Can you work these out from the model? Positions are in its coordinate system, mm. Face numbers are marked on the shaded views. A direction names the side the tool comes from. Give positions to 0.01 mm unless a question says otherwise; leave off trailing zeros. Order: outer loops, then holes, each group sorted by start corner. A loop starts at its lowest first (then second) coordinate and runs counter-clockwise, first axis right, second up. Notation, with made-up numbers: (17.25, 82.5) - (65.25, 82.5) arc R30 cw to (65.25, 112.5) - close; hole circle Ø1 at (-16.5, -23). An arc over 180 degrees is marked (long way). Return JSON: item names as keys, results as strings.
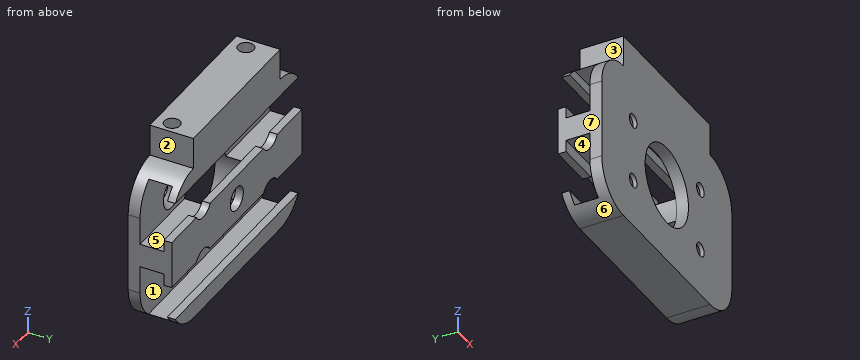
```python
from build123d import *
from build123d.topology import SkipClean

# Parameters (mm, degrees)
SKETCH1_R           = 9.999999259
SKETCH1_R_2         = 1.748202303
SKETCH1_R_3         = 1.748202071
BOSS_EXTRUDE1_DEPTH = 3
BOSS_EXTRUDE2_REACH = 65.317
BOSS_EXTRUDE3_DEPTH = 59.999998659
CUT_EXTRUDE1_START  = 18
SKETCH3_R           = 9.999999259
CUT_EXTRUDE1_DEPTH  = 18
SKETCH4_W           = 63.792856733
SKETCH4_H           = 41.767533566
CUT_EXTRUDE2_DEPTH  = 29
SKETCH5_R           = 2.99999956
CUT_EXTRUDE3_DEPTH  = 29
CHAMFER1_SIZE       = 2
CHAMFER2_SIZE       = 2
SKETCH6_R           = 3.748202071
SKETCH6_R_2         = 3.748202303
CUT_EXTRUDE4_DEPTH  = 3
SKETCH7_R           = 1.5
CUT_EXTRUDE5_DEPTH  = 2
SKETCH9_W           = 40.000000969
SKETCH9_H           = 2
BOSS_EXTRUDE4_DEPTH = 11
SKETCH10_W          = 40.000000969
SKETCH10_H          = 10.999999914
SKETCH10_R          = 2
BOSS_EXTRUDE5_DEPTH = 6
CUT_EXTRUDE6_START  = -3.945921595
SKETCH10_3_R        = 2
CUT_EXTRUDE6_DEPTH  = 3.945921595


with BuildPart() as part:
    # Sketch1 → Boss-Extrude1 (new body)
    with BuildSketch(Plane(origin=(0, 0, 0), x_dir=(1, 0, 0), z_dir=(0, 1, 0))):
        with BuildLine():
            Line((-19.999999553, -20.000000484), (20.000001416, -20.000000484))
            ThreePointArc((20.000001416, -20.000000484), (27.071068604, -17.071068441), (29.999999329, -10.000000708))
            Line((29.999999329, -10.000000708), (29.999999329, 9.999998845))
            ThreePointArc((29.999999329, 9.999998845), (27.071068411, 17.071066386), (20.000001416, 19.999998622))
            Line((20.000001416, 19.999998622), (-19.999999553, 19.999998622))
            ThreePointArc((-19.999999553, 19.999998622), (-27.071067207, 17.071066499), (-29.999999329, 9.999998845))
            Line((-29.999999329, 9.999998845), (-29.999999329, -10.000000708))
            ThreePointArc((-29.999999329, -10.000000708), (-27.071067207, -17.071068362), (-19.999999553, -20.000000484))
        make_face()
        with Locations(Location((0, 0, 0), (0, 0, 270))):
            Circle(SKETCH1_R, mode=Mode.SUBTRACT)
        with Locations(Location((15.500057023, 8.001796436, 0), (0, 0, 270))):
            Circle(SKETCH1_R_2, mode=Mode.SUBTRACT)
        with Locations(Location((-15.500057023, 8.001796436, 0), (0, 0, 270))):
            Circle(SKETCH1_R_2, mode=Mode.SUBTRACT)
        with Locations(Location((-15.500057023, -7.998204092, 0), (0, 0, 270))):
            Circle(SKETCH1_R_3, mode=Mode.SUBTRACT)
        with Locations(Location((15.500057023, -7.998204092, 0), (0, 0, 270))):
            Circle(SKETCH1_R_3, mode=Mode.SUBTRACT)
    extrude(amount=BOSS_EXTRUDE1_DEPTH)

    # Boss-Extrude2: up to this face of the body (flat: up to its plane)
    boss_extrude2_end = Plane(part.part.faces().sort_by_distance((-29.999999329, 1.5, 9.31e-07))[0])
    # Sketch2 → Boss-Extrude2 (add, up to the picked face)
    with BuildSketch(Plane(origin=(29.999999329, 0, 0), x_dir=(0, 0, -1), z_dir=(1, 0, 0)), mode=Mode.PRIVATE) as boss_extrude2_sk1:
        Polygon((-6.054078553, 8.999999586), (-3.054078061, 8.999999586), (-3.054078061, 3), (2.94592106, 3), (2.94592106, 8.999999586), (5.945921552, 8.999999586), (5.945921552, 10.999999914), (-6.054078553, 10.999999914), align=None)
    boss_extrude2_tool1 = split(extrude(boss_extrude2_sk1.sketch, amount=-BOSS_EXTRUDE2_REACH, mode=Mode.PRIVATE), bisect_by=boss_extrude2_end, keep=Keep.BOTH, mode=Mode.PRIVATE)
    # Sketch2 → Boss-Extrude2 (add, up to the picked face)
    with BuildSketch(Plane(origin=(29.999999329, 0, 0), x_dir=(0, 0, -1), z_dir=(1, 0, 0)), mode=Mode.PRIVATE) as boss_extrude2_sk2:
        Polygon((-15.554079178, 10.999999914), (-20.000000484, 10.999999914), (-20.000000484, 3), (-18.05407889, 3), (-18.05407889, 8.999999586), (-15.554079178, 8.999999586), align=None)
    boss_extrude2_tool2 = split(extrude(boss_extrude2_sk2.sketch, amount=-BOSS_EXTRUDE2_REACH, mode=Mode.PRIVATE), bisect_by=boss_extrude2_end, keep=Keep.BOTH, mode=Mode.PRIVATE)
    # Sketch2 → Boss-Extrude2 (add, up to the picked face)
    with BuildSketch(Plane(origin=(29.999999329, 0, 0), x_dir=(0, 0, -1), z_dir=(1, 0, 0)), mode=Mode.PRIVATE) as boss_extrude2_sk3:
        Polygon((19.737818007, 10.999999914), (15.445922178, 10.999999914), (15.445922178, 8.999999586), (17.945919793, 8.999999586), (17.945919793, 3), (19.872933217, 3), (19.872933217, 8.999999586), (19.737818007, 8.999999586), align=None)
    boss_extrude2_tool3 = split(extrude(boss_extrude2_sk3.sketch, amount=-BOSS_EXTRUDE2_REACH, mode=Mode.PRIVATE), bisect_by=boss_extrude2_end, keep=Keep.BOTH, mode=Mode.PRIVATE)
    add(boss_extrude2_tool1.solids().sort_by(Axis((29.999999, 7.6, 0.054079), (-1, 0, 0)))[0])
    add(boss_extrude2_tool2.solids().sort_by(Axis((29.999999, 7.72931, 18.48663), (-1, 0, 0)))[0])
    add(boss_extrude2_tool3.solids().sort_by(Axis((29.999999, 7.704328, -18.348039), (-1, 0, 0)))[0])

    # Sketch2<3> → Boss-Extrude3 (add)
    with BuildSketch(Plane(origin=(29.999999329, 0, 0), x_dir=(0, 0, -1), z_dir=(1, 0, 0))):
        Polygon((19.945920121, 10.999999914), (19.737818007, 10.999999914), (19.737818007, 8.999999586), (19.872933217, 8.999999586), (19.945920121, 8.999999586), align=None)
        Polygon((19.999998622, 10.999999914), (19.945920121, 10.999999914), (19.945920121, 8.999999586), (19.872933217, 8.999999586), (19.872933217, 3), (19.999998622, 3), align=None)
    extrude(amount=-BOSS_EXTRUDE3_DEPTH)

    # Sketch3 → Cut-Extrude1 (cut)
    with SkipClean():  # the faces are left unmerged after this step: merging them gives an invalid solid
        with BuildSketch(Plane.XZ.offset(-8.999999586).offset(CUT_EXTRUDE1_START)):
            with Locations(Location((0, 0, 0), (0, 0, 342.86691881))):
                Circle(SKETCH3_R)
        extrude(amount=-CUT_EXTRUDE1_DEPTH, mode=Mode.SUBTRACT)
    add(part.part.scale(1), mode=Mode.REPLACE)  # the faces are merged on a copy

    # Sketch4 → Cut-Extrude2 (cut)
    with BuildSketch(Plane.XZ):
        with Locations((1.275857135, -0.402901322)):
            Rectangle(SKETCH4_W, SKETCH4_H)
        with BuildLine():
            Line((20.000001416, 20.000000484), (-19.999999553, 20.000000484))
            ThreePointArc((-19.999999553, 20.000000484), (-27.071067207, 17.071068362), (-29.999999329, 10.000000708))
            Line((-29.999999329, 10.000000708), (-29.999999329, -9.999998845))
            ThreePointArc((-29.999999329, -9.999998845), (-27.071067207, -17.071066499), (-19.999999553, -19.999998622))
            Line((-19.999999553, -19.999998622), (20.000001416, -19.999998622))
            ThreePointArc((20.000001416, -19.999998622), (27.071068411, -17.071066386), (29.999999329, -9.999998845))
            Line((29.999999329, -9.999998845), (29.999999329, 10.000000708))
            ThreePointArc((29.999999329, 10.000000708), (27.071068604, 17.071068441), (20.000001416, 20.000000484))
        make_face(mode=Mode.SUBTRACT)
    extrude(amount=-CUT_EXTRUDE2_DEPTH, mode=Mode.SUBTRACT)

    # Sketch5 → Cut-Extrude3 (cut)
    with BuildSketch(Plane(origin=(0, 10.999999914, 0), x_dir=(1, 0, 0), z_dir=(0, 1, 0))):
        with Locations(Location((0, 0, 0), (0, 0, 270))):
            Circle(SKETCH5_R)
    extrude(amount=-CUT_EXTRUDE3_DEPTH, mode=Mode.SUBTRACT)

    # Chamfer1
    chamfer1_edges = [part.edges().sort_by_distance(p)[0] for p in [
        (-15.500057023, 3, 6.250002021),
    ]]
    chamfer(chamfer1_edges, length=CHAMFER1_SIZE)

    # Chamfer2
    chamfer2_edges = [part.edges().sort_by_distance(p)[0] for p in [
        (15.500057023, 3, -9.749998739),
        (-15.500057023, 3, -9.749998739),
        (15.500057023, 3, 6.250002021),
    ]]
    chamfer(chamfer2_edges, length=CHAMFER2_SIZE)

    # Sketch6 → Cut-Extrude4 (cut)
    with BuildSketch(Plane(origin=(0, 10.999999914, 0), x_dir=(1, 0, 0), z_dir=(0, 1, 0))):
        with Locations((-15.500057023, -7.998204092)):
            Circle(SKETCH6_R)
        with Locations((-15.500057023, 8.001796436)):
            Circle(SKETCH6_R_2)
        with Locations((15.500057023, -7.998204092)):
            Circle(SKETCH6_R)
        with Locations((15.500057023, 8.001796436)):
            Circle(SKETCH6_R_2)
    extrude(amount=-CUT_EXTRUDE4_DEPTH, mode=Mode.SUBTRACT)

    # Sketch7 → Cut-Extrude5 (cut)
    with BuildSketch(Plane.XY.offset(20.000000484)):
        with Locations((-17, 3.999999914)):
            Circle(SKETCH7_R)
        with Locations((17, 3.999999914)):
            Circle(SKETCH7_R)
    extrude(amount=-CUT_EXTRUDE5_DEPTH, mode=Mode.SUBTRACT)

    # Sketch9 → Boss-Extrude4 (add)
    with BuildSketch(Plane(origin=(0, 10.999999914, 0), x_dir=(1, 0, 0), z_dir=(0, 1, 0))):
        with Locations((9.31e-07, -21.000000484)):
            Rectangle(SKETCH9_W, SKETCH9_H)
    extrude(amount=-BOSS_EXTRUDE4_DEPTH)

    # Sketch10 → Boss-Extrude5 (add)
    with BuildSketch(Plane.XY.offset(22.000000484)):
        with Locations((9.31e-07, 5.499999957)):
            Rectangle(SKETCH10_W, SKETCH10_H)
        with Locations((-17, 3.999999914)):
            Circle(SKETCH10_R, mode=Mode.SUBTRACT)
        with Locations((17, 3.999999914)):
            Circle(SKETCH10_R, mode=Mode.SUBTRACT)
    extrude(amount=BOSS_EXTRUDE5_DEPTH)

    # Sketch10<3> → Cut-Extrude6 (cut)
    with BuildSketch(Plane.XY.offset(22.000000484).offset(CUT_EXTRUDE6_START)):
        with Locations(Location((17, 3.999999914, 0), (0, 0, 209.999997166))):
            Circle(SKETCH10_3_R)
        with Locations(Location((-17, 3.999999914, 0), (0, 0, 209.999997166))):
            Circle(SKETCH10_3_R)
    extrude(amount=CUT_EXTRUDE6_DEPTH, mode=Mode.SUBTRACT)


solid = part.part
```
1. Suppose I cut it at D-D (z = 8). State how many separate pieces and enclosed holes the cut face has, plus the area to 3 significant figures.
Checks:
{"separate pieces": "4", "enclosed holes": "0", "area": "115 mm^2"}
2. Suppose I cut it at A-A (x = 0). List the corners of the cut face in (y, z) for me.
Checks:
{"outline": "(0, -20) - (11, -20) - (11, -15.45) - (9, -15.45) - (9, -17.95) - (3, -17.95) - (3, -10) - (0, -10) - close; (0, 10) - (3, 10) - (3, 18.05) - (9, 18.05) - (9, 15.55) - (11, 15.55) - (11, 28) - (0, 28) - close; (9, -5.95) - (11, -5.95) - (11, -3) - (9, -3) - close; (9, 3) - (11, 3) - (11, 6.05) - (9, 6.05) - close"}
3. For pin 1 Ø2.5 at (x, z) = (-13, -17) entering from -Y; pin 2 Ø4 at (x, z) = (1.5, 8.5) entering from +Y; pin 3 Ø4 at (y, z) = (5.5, 25) entering from -X; pin 4 Ø5.5 at (x, z) = (15.5, 8) entering from +Y, each with a flat end and sliding along its axis, tell me the tip position at first contact or that it passes through.
Checks:
{"pin 1": "y = 0", "pin 2": "y = 3", "pin 3": "x = -20", "pin 4": "y = 2"}
4. Suppose I cut it at B-B (z = 0). List the corners of the cut face in (x, y) for me, plus the area to 3 significant figures.
Checks:
{"outline": "(-30, 0) - (-10, 0) - (-10, 9) - (-3, 9) - (-3, 11) - (-30, 11) - close; (3, 9) - (10, 9) - (10, 0) - (30, 0) - (30, 11) - (3, 11) - close", "area": "468 mm^2"}
5. On a 3-axis mill with a long thin cutter (end or side, diameter ignored), from which of +Z, -Z, +X, -X, +Y, -Y can I reach the whole of each face in a straight line? I mean the marked faces 1, 2 and 3. Say none if no direction works.
Checks:
{"face 1": "+X, -X", "face 2": "+Z, +X, +Y, -Y", "face 3": "+Z, -X, +Y, -Y"}
6. Thinking about a two-plate mould opening in Z: for the marked faces 4, 5, 6 and 7, which applies, +Z half, -Z half, draft (parallel to the pull), parting line (faces both ways), or undercut?
Checks:
{"face 4": "undercut", "face 5": "undercut", "face 6": "-Z half", "face 7": "draft"}
7. Suppose I cut it at C-C (x = 7). List the corners of the cut face in (y, z) for me.
Checks:
{"outline": "(0, -20) - (11, -20) - (11, -15.45) - (9, -15.45) - (9, -17.95) - (3, -17.95) - (3, -7.14) - (0, -7.14) - close; (0, 7.14) - (3, 7.14) - (3, 18.05) - (9, 18.05) - (9, 15.55) - (11, 15.55) - (11, 28) - (0, 28) - close; (9, -5.95) - (11, -5.95) - (11, 6.05) - (9, 6.05) - close"}
8. If I drill on L1, parallel to Z at x = 7.5, y = 10.25; L2, parallel to Z at x = 15.5, y = 9.25; L3, parallel to Y at x = 16, z = 16, over which ranges is the centre line in solid material (lowest first)? Write a range as [from, to].
Checks:
{"L1": "[-20, -15.45], [-5.95, 6.05], [15.55, 28]", "L2": "[-20, -15.45], [-4.25, 4.25], [15.55, 28]", "L3": "[0, 3], [9, 11]"}
